Geometry: see drawing. Coordinates: mm, zero at the bounding-box minimum. Give positions to 0.01 mm unless a question says otherwise; leave off trailing zeros. Write each loop counter-clockwise with the first axis right and the second up, starting at its lowest first coordinate (ties: lowest second). Pieces come first, ordered by that corner, then holes. Notation, with made-up numbers: M 67,-29.5 L 121,-29.5 A7 ccw 121,-24.5 Z; hole C 79,-30 d4. An arc over 180 degrees is marked long. Use one line per item in the form item = value. Start each with the question number.
Item 1: Material intervals for line 1 along Z through (x, y) = (5, 1.75) (1 decimal); line 2 along Z through (x, y) = (25.5, 4.15), sorted ascending. Write a range as from..to.
Item 2: Section query C-C on x = 19. Return loops of the section in (y, z) (1 decimal).
Item 3: Section query B-B on y = 4. Return loops of the section in (x, z).
Item 4: Section query A-A on x = 5. Return loops of the section in (y, z) (1 decimal).
Item 5: Contact query for flat-ended pins moving along their axis: P1, Ø2, axis at x = 11, y = 1, coming from the +Z side; P2, Ø3, axis at x = 24, z = 25.5, coming from the +Y side; P3, Ø5, axis at x = 18, z = 24.5, coming from the -Y side; P4, Ø3, axis at x = 5, z = 25, coming from the -Y side. Output: stop coordinate, or through.
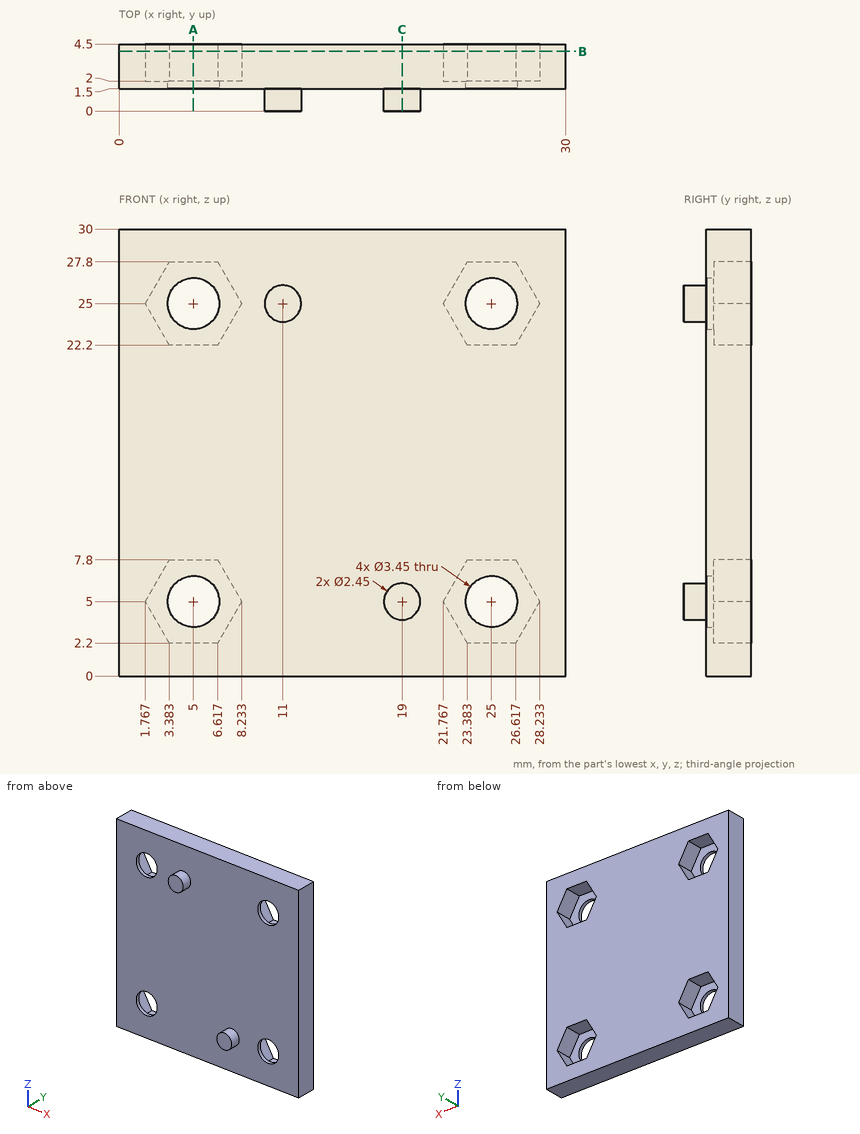
Answer sheet:
q1.line_1 = 0..3.3, 6.7..23.3, 26.7..30
q1.line_2 = 0..2.2, 7.8..22.2, 27.8..30
q2.outline = M 0,3.8 L 1.5,3.8 L 1.5,0 L 4.5,0 L 4.5,30 L 1.5,30 L 1.5,6.2 L 0,6.2 Z
q3.outline = M 0,0 L 30,0 L 30,30 L 0,30 Z; hole M 1.77,5 L 3.38,2.2 L 6.62,2.2 L 8.23,5 L 6.62,7.8 L 3.38,7.8 Z; hole M 1.77,25 L 3.38,22.2 L 6.62,22.2 L 8.23,25 L 6.62,27.8 L 3.38,27.8 Z; hole M 21.77,5 L 23.38,2.2 L 26.62,2.2 L 28.23,5 L 26.62,7.8 L 23.38,7.8 Z; hole M 21.77,25 L 23.38,22.2 L 26.62,22.2 L 28.23,25 L 26.62,27.8 L 23.38,27.8 Z
q4.outline = M 1.5,0 L 4.5,0 L 4.5,2.2 L 2,2.2 L 2,3.3 L 1.5,3.3 Z; M 1.5,6.7 L 2,6.7 L 2,7.8 L 4.5,7.8 L 4.5,22.2 L 2,22.2 L 2,23.3 L 1.5,23.3 Z; M 1.5,26.7 L 2,26.7 L 2,27.8 L 4.5,27.8 L 4.5,30 L 1.5,30 Z
q5.P1 = 30
q5.P2 = 2
q5.P3 = 1.5
q5.P4 = through
